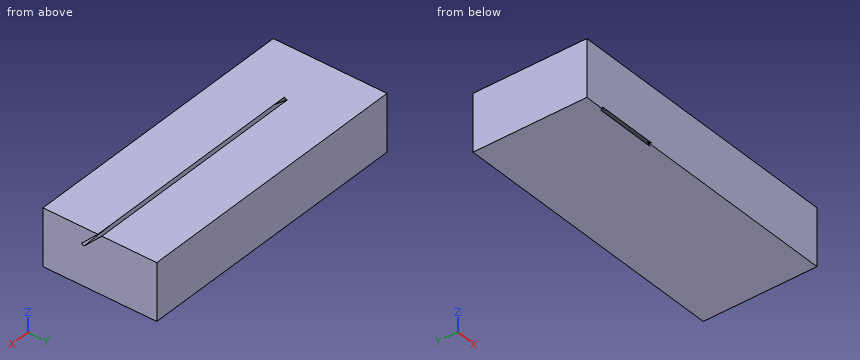
from build123d import *

# Parameters (mm, degrees)
SKETCH1_W           = 50
SKETCH1_H           = 20
BOSS_EXTRUDE1_DEPTH = 10
CUT_EXTRUDE1_DEPTH  = 0.25


with BuildPart() as part:
    # Sketch1 → Boss-Extrude1 (new body)
    with BuildSketch(Plane.XY):
        Rectangle(SKETCH1_W, SKETCH1_H)
    extrude(amount=BOSS_EXTRUDE1_DEPTH)

    # Sketch2 → Cut-Extrude1 (cut, symmetric)
    with BuildSketch(Plane(origin=(0, -5, 5), x_dir=(1, 0, 0), z_dir=(0, -0.707106781, 0.707106781))):
        Polygon((-23, -10.071067812), (35.375550351, 5.570613762), (29.163893269, 28.752833593), (-10.439065609, 18.141252744), align=None)
    extrude(amount=CUT_EXTRUDE1_DEPTH, both=True, mode=Mode.SUBTRACT)


solid = part.part
Model file for the job. Use its own axes, mm. Give positions to 0.01 mm unless a question says otherwise; leave off trailing zeros. Order: outer loops, then holes, each group sorted by start corner. A loop starts at its lowest first (then second) coordinate and runs counter-clockwise, first axis right, second up. Notation, with made-up numbers: M -8,7 L 37,7 A18 cw 37,23 Z; hole C 15,26 d2. An arc over 180 degrees is marked long. Put each result on its own line as item: value. Start each with the question number.
(1) Band-saw the part on B-B on z = 4.75. Give the cut face in (x, y).
(2) Drill centre lines: L1, parallel to Z at x = 11.5, y = -3.25; L2, parallel to Z at x = 13, y = -2.5; L3, parallel to Y at x = -10.5, z = 9. Where is each one in solid material? Low to high. Write a range as [from, to].
(3) Band-saw the part on D-D on z = 8.25. Give the cut face in (x, y), then the cut area to 3 significant figures.
(4) Band-saw the part on A-A on y = -8.25. Give the cut face in (x, z).
(5) Band-saw the part on C-C on x = -17.5. Give the cut face in (y, z).
(6) Pin check, flat tip, straight feed: pin 1 Ø6 at (x, y) = (13, -0.5) entering from -Z. Stop position of the tip, or through.
Results below:
1. outline: M -25,-10 L 25,-10 L 25,10 L -25,10 Z; hole M -18.78,-5.6 L 12.33,-5.6 L 14.2,-4.9 L -18.56,-4.9 Z
2. L1: z = [0, 6.4], [7.1, 10]
2. L2: z = [0, 7.15], [7.85, 10]
2. L3: y = [-10, -1.35], [-0.65, 10]
3. outline: M -25,-10 L 25,-10 L 25,-2.1 L -16.58,-2.1 L -16.36,-1.4 L 25,-1.4 L 25,10 L -25,10 Z
3. area: 971 mm2
4. outline: M -25,0 L 25,0 L 25,10 L -25,10 Z; hole M -20.67,1.4 L -3.5,1.4 L -1.63,2.1 L -20.45,2.1 Z
5. outline: M -10,0.35 L -3.56,6.79 L -3.21,6.44 L -9.65,0 L 10,0 L 10,10 L -10,10 Z
6. pin 1: stops at z = 0
